Read the model definition and answer for the solid it produces. Units are mm, in the model's axes. A direction names the side the tool comes from. Coordinates: 2 decimals unless noted, no trailing zeros. Order: outer loops, then holes, each group sorted by start corner. A loop starts at its lowest first (then second) coordinate and runs counter-clockwise, first axis right, second up. Notation, with made-up numbers: (71.5, 44) - (127.5, 44) arc R20 cw to (127.5, 63) - close; hole circle Ø7 at (-2, 29). An arc over 180 degrees is marked (long way). Use one line per item in the form item = value.
Autodesk Inventor part; units mm, degrees
ref_plane "YZ Plane" through (0, 0, 0) normal (1, 0, 0) x (0, 1, 0)
ref_plane "XZ Plane" through (0, 0, 0) normal (0, 1, 0) x (-1, 0, 0)
ref_plane "XY Plane" through (0, 0, 0) normal (0, 0, 1) x (1, 0, 0)
sketch "草图1" plane through (0, 0, 0) normal (0, 0, 1) x (1, 0, 0)
  line L0 (-13, 9) -> (13, 9)
  line L1 (13, 9) -> (13, -9)
  line L2 (13, -9) -> (-13, -9)
  line L3 (-13, -9) -> (-13, 9)
  line L4 (-13, 9) -> (13, -9) construction
  line L5 (13, 9) -> (-13, -9) construction
  point P0 (0, 0)
  dimension "d0" = 26
  dimension "d1" = 18
extrude "拉伸1" add sketch "草图1" along normal blind 13
sketch "草图2" plane through (0, 0, 13) normal (0, 0, 1) x (1, 0, 0)
  line L0 (13, 9) -> (-13, 9)
  line L1 (13, -9) -> (13, 9)
  line L2 (-13, 9) -> (13, 9)
  line L3 (13, 9) -> (13, -3)
  line L4 (13, -3) -> (-13, -3)
  line L5 (-13, -3) -> (-13, 9)
  arc A0 (-10, 9) -> (10, 9) centre (0, 9) ccw
  point P0 (0, 0)
  point P1 (10, 9)
  dimension "d4" = 12
  dimension "d5" = 20
extrude "拉伸2" add sketch "草图2" along normal blind 7 contours L1 L4 L5 L0 A0
sketch "草图3" plane through (0, 0, 13) normal (0, 0, 1) x (1, 0, 0)
  line L0 (10, 9) -> (-10, 9)
  arc A0 (-5, 9) -> (5, 9) centre (0, 9) ccw
  point P0 (0, 0)
  dimension "d8" = 10
extrude "拉伸3" cut sketch "草图3" against normal blind 13
properties part number "2-4"
(1) Given pin 1 Ø5 at (x, y) = (1, 5.5) entering from +Z, flat-ended and moving along its own axis, determine where the tip first touches the part or whether it passes through.
Answer list:
pin_1 = 13
(2) Section D-D, the plane y = 0 is taken. Write down the section's boundary in (x, z).
Answer list:
outline = (-13, 0) - (13, 0) - (13, 20) - (4.36, 20) - (4.36, 13) - (-4.36, 13) - (-4.36, 20) - (-13, 20) - close
(3) Section B-B, the plane z = 9.5 is taken. Write down the section's boundary in (x, y).
Answer list:
outline = (-13, -9) - (13, -9) - (13, 9) - (5, 9) arc R5 cw to (-5, 9) - (-13, 9) - close
(4) Which of the six approach directions +Z, -Z, +X, -X, +Y, -Y give full straight-line access (tool end or side, diameter ignored) to faces 4 (the flat face through (0, -6, 13)), 5 (the cylindrical face through (0, -1, 16)), 6 (the flat face through (9, 9, 8))?
Answer list:
face_4 = +Z, +X, -X, -Y
face_5 = +Z, +Y
face_6 = +Z, -Z, +X, -X, +Y
(5) Straight lines are drawn through the part: L1, parallel to Y at x = 0, z = 6.5; L2, parallel to Z at x = -9.5, y = -5.75; L3, parallel to X at y = 6.5, z = 19. For each, find the intervals that lie inside material, in ascending order.
Answer list:
L1 = -9 to 4
L2 = 0 to 13
L3 = -13 to -9.68, 9.68 to 13
(6) The mould has two halves that part along X. Classify faces 1 (the flat face through (0, 3, 13)), 2 (the flat face through (0, -9, 6)), 3 (the flat face through (-13, 0, 10)): +X half, -X half, draft (parallel to the pull), parting line (faces both ways), or undercut.
Answer list:
face_1 = undercut
face_2 = draft
face_3 = -X half
(7) Section C-C, the plane x = 0 is taken. Write down the section's boundary in (y, z).
Answer list:
outline = (-9, 0) - (4, 0) - (4, 13) - (-1, 13) - (-1, 20) - (-3, 20) - (-3, 13) - (-9, 13) - close
(8) Section A-A, the plane y = 7.5 is taken. Write down the section's boundary in (x, z).
Answer list:
outline = (-13, 0) - (-4.77, 0) - (-4.77, 13) - (-9.89, 13) - (-9.89, 20) - (-13, 20) - close; (4.77, 0) - (13, 0) - (13, 20) - (9.89, 20) - (9.89, 13) - (4.77, 13) - close
